Design review of the part shown in the three views and the two pictorial views. Dimensions are in mm from the part's minimum x, y and z. A direction names the side the tool comes from. Coordinates: 2 decimals unless noted, no trailing zeros. Loops run counter-clockwise (first coordinate to the right, second up) from the corner with the lowest first, then second, coordinate; pieces in that order, holes last. Notation, with made-up numbers: M 28,77 L 51,77 A22 cw 51,102 Z; hole C 70.5,-11.5 d7. An arc over 180 degrees is marked long. Answer as a JSON object with one key per item and string values. Group by question number.
Item 1: Add section A-A (y = 27). State the section outline as (x, z) points (1 decimal).
Item 2: Tool access review of the marked faces 1 and 2: name each direction out of +Z, -Z, +X, -X, +Y, -Y from which nothing blocks a thin tool from reaching the whole face with its end or side.
Item 3: Add section D-D (y = 20). State the section outline as (x, z) points (1 decimal).
Item 4: Insertion check: pin 1 (4 mm diameter, centred on x = 46, z = 23.5, fed in from +Y); pin 2 (4 mm diameter, centred on x = 53.5, z = 15, fed in from -Y); pin 3 (1.8 mm diameter, centred on x = 3.025, z = 8.26, fed in from +Y); pin 4 (3.5 mm diameter, centred on x = 3.86, y = 20, fed in from -Z). Each pin has a flat end and moves straight along its axis. Give the tip position at first contact, or say it passes through.
Item 5: Add section B-B (x = 28). State the section outline as (y, z) points (1 decimal).
Item 6: Add section C-C (z = 8.26). State the section outline as (x, y) points (1 decimal).
Item 7: Wall thickness on L1, parallel to X at y = 39.75, z = 8.26 (1 decimal); L2, parallel to X at y = 39.5, z = 6.75 (1 decimal); L3, parallel to Y at x = 28, z = 26 (1 decimal): over which ranges is each line inside the solid? List them lowest first. Write a range as from..to.
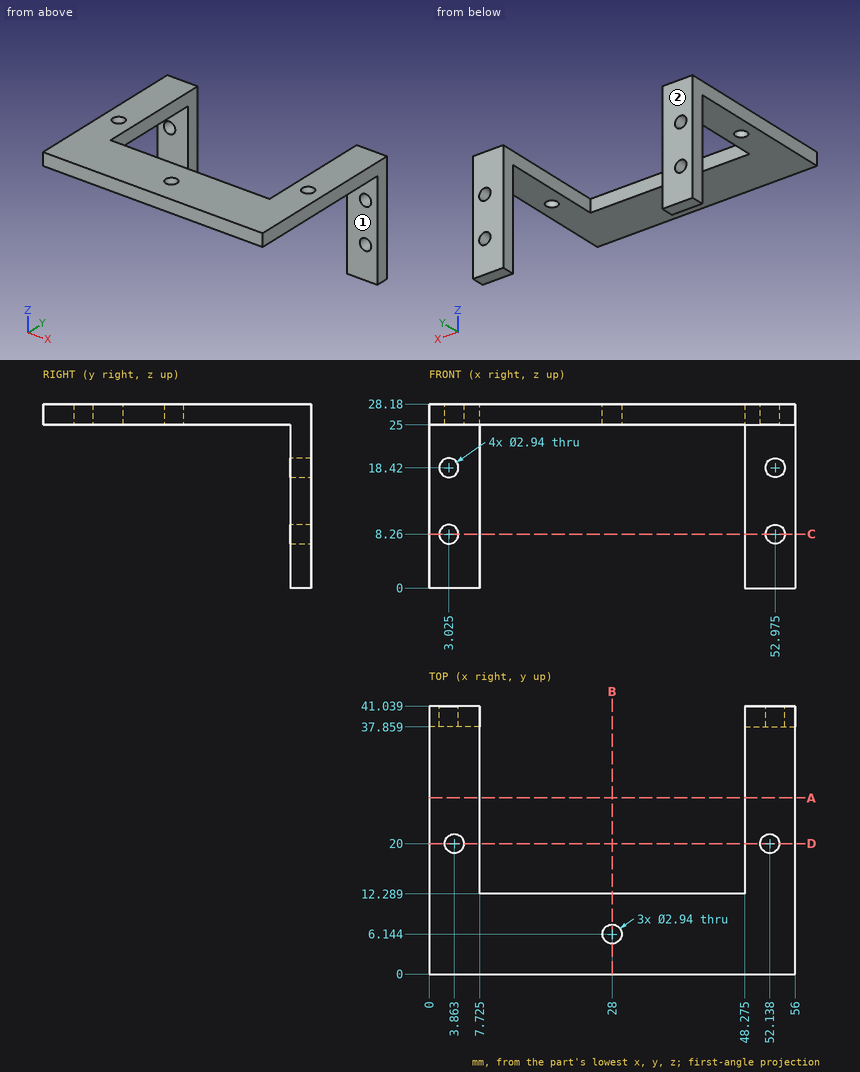
From the geometry:
{
 "1": {"outline": "M 0,25 L 7.7,25 L 7.7,28.2 L 0,28.2 Z; M 48.3,25 L 56,25 L 56,28.2 L 48.3,28.2 Z"},
 "2": {"face 1": "-Z, +X, -X, -Y", "face 2": "+Z, -Z, +X, -X, +Y"},
 "3": {"outline": "M 0,25 L 2.4,25 L 2.4,28.2 L 0,28.2 Z; M 5.3,25 L 7.7,25 L 7.7,28.2 L 5.3,28.2 Z; M 48.3,25 L 50.7,25 L 50.7,28.2 L 48.3,28.2 Z; M 53.6,25 L 56,25 L 56,28.2 L 53.6,28.2 Z"},
 "4": {"pin 1": "stops at y = 12.29", "pin 2": "stops at y = 37.86", "pin 3": "passes through", "pin 4": "stops at z = 25"},
 "5": {"outline": "M 0,25 L 4.7,25 L 4.7,28.2 L 0,28.2 Z; M 7.6,25 L 12.3,25 L 12.3,28.2 L 7.6,28.2 Z"},
 "6": {"outline": "M 0,37.9 L 1.6,37.9 L 1.6,41 L 0,41 Z; M 4.5,37.9 L 7.7,37.9 L 7.7,41 L 4.5,41 Z; M 48.3,37.9 L 51.5,37.9 L 51.5,41 L 48.3,41 Z; M 54.4,37.9 L 56,37.9 L 56,41 L 54.4,41 Z"},
 "7": {"L1": "x = 0..1.6, 4.5..7.7, 48.3..51.5, 54.4..56", "L2": "x = 0..7.7, 48.3..56", "L3": "y = 0..4.7, 7.6..12.3"}
}
